Part model, mm, in its own coordinate system. Give positions to 0.01 mm unless a question says otherwise; leave off trailing zeros. Order: outer loops, then holes, each group sorted by start corner. A loop starts at its lowest first (then second) coordinate and runs counter-clockwise, first axis right, second up. Notation, with made-up numbers: (13, -3) -> (48, -3) arc R29 cw to (48, 30) -> close; hole circle Ø11 at (42.25, 86). An arc over 180 degrees is marked (long way). Write item = value, one per line. Start each with the question number.
(1) Saw through at C-C, the plane y = 7. List the corners of the cut face in (x, z), then the cut area to 3 significant figures.
(2) Saw through at D-D, the plane x = 48. List the corners of the cut face in (y, z).
(3) Flat gauge pins, fed straight in: pin 1 (8.5 mm diameter, centred on x = 4, z = -1.5, fed in from -Y); pin 2 (1 mm diameter, centred on x = -12, y = -14, fed in from -Z); pin 3 (12 mm diameter, centred on y = -88, z = 1, fed in from -X) (3 decimals); pin 4 (1 mm diameter, centred on x = 9, y = -63.5, fed in from -Z). Where does each tip first touch, or does it go through?
(4) Probe line 1 along X through (y, z) = (-26, 0) (3 decimals); line 2 along Y through (x, z) = (0, -9); line 3 along Y through (x, z) = (-49, -5). List the from-to ranges inside material, lowest first. Write a range as from..to.
(5) Saw through at B-B, the plane z = -36. List the corners of the cut face in (x, y).
(6) Two-plate mould, pull along Z, no slides. Class faces 1 (the flat face through (21, 0, -1)), 2 (the cylindrical face through (9.085, -50.089, 2.861)), 3 (the cylindrical face through (8.24, -50.09, 2.59)): pulls with the +Z half, pulls with the -Z half, needs draft (parallel to the pull), parting line crosses it, or undercut.
from build123d import *

# Parameters (mm, degrees)
SKETCH1_R               = 101.6
BOSS_EXTRUDE1_DEPTH     = 25.4
SKETCH2_R               = 9.525
SKETCH2_R_2             = 8.636
BOSS_EXTRUDE2_DEPTH     = 101.6
SKETCH3_R               = 2.38125
CUT_EXTRUDE1_DEPTH      = 102.6
CUT_EXTRUDE1_DEPTH_BACK = 102.6
CUT_EXTRUDE2_DEPTH      = 25.908
CUT_EXTRUDE2_DEPTH_BACK = 25.4


with BuildPart() as part:
    # Sketch1 → Boss-Extrude1 (new body)
    with BuildSketch(Plane(origin=(0, 0, 0), x_dir=(1, 0, 0), z_dir=(0, 1, 0))):
        Circle(SKETCH1_R)
    extrude(amount=BOSS_EXTRUDE1_DEPTH)

    # Sketch2 → Boss-Extrude2 (add)
    with BuildSketch(Plane.XZ):
        Circle(SKETCH2_R)
        Circle(SKETCH2_R_2, mode=Mode.SUBTRACT)
    extrude(amount=BOSS_EXTRUDE2_DEPTH)

    # Sketch3 → Cut-Extrude1 (cut, two sides)
    with BuildSketch(Plane.XY) as cut_extrude1_sk:
        with Locations((0, -12.7)):
            Circle(SKETCH3_R)
    extrude(amount=CUT_EXTRUDE1_DEPTH, mode=Mode.SUBTRACT)
    extrude(cut_extrude1_sk.sketch, amount=-CUT_EXTRUDE1_DEPTH_BACK, mode=Mode.SUBTRACT)

    # Sketch4 → Cut-Extrude2 (cut, two sides)
    with BuildSketch(Plane(origin=(0, 0, 0), x_dir=(0, 0, -1), z_dir=(1, 0, 0))) as cut_extrude2_sk:
        with BuildLine():
            Line((-1.5875, -82.55), (-1.5875, -57.15))
            ThreePointArc((-1.5875, -57.15), (0, -55.5625), (1.5875, -57.15))
            Line((1.5875, -57.15), (1.5875, -82.55))
            ThreePointArc((1.5875, -82.55), (0, -84.1375), (-1.5875, -82.55))
        make_face()
    extrude(amount=CUT_EXTRUDE2_DEPTH, mode=Mode.SUBTRACT)
    extrude(cut_extrude2_sk.sketch, amount=-CUT_EXTRUDE2_DEPTH_BACK, mode=Mode.SUBTRACT)


solid = part.part
Results list:
q1.outline = circle Ø203.2 at (0, 0)
q1.area = 32,400 mm^2
q2.outline = (0, -89.55) -> (25.4, -89.55) -> (25.4, 89.55) -> (0, 89.55) -> close
q3.pin_1 = 0
q3.pin_2 = through
q3.pin_3 = -9.525
q3.pin_4 = -4.3
q4.line_1 = -9.525..-8.636, 8.636..9.525
q4.line_2 = -101.6..-15.08, -10.32..25.4
q4.line_3 = 0..25.4
q5.outline = (-95.01, 0) -> (95.01, 0) -> (95.01, 25.4) -> (-95.01, 25.4) -> close
q6.face_1 = needs draft
q6.face_2 = parting line crosses it
q6.face_3 = undercut
